Check sheet for the modelled part. Datum: model origin and axes. Units: mm. Face numbers are marked on the shaded views. A direction names the side the tool comes from. Round coordinates to 2 decimals unless told otherwise and drop trailing zeros. Write each loop counter-clockwise with the first axis right and the second up, starting at its lowest first coordinate (ties: lowest second). Pieces come first, ordered by that corner, then holes. Notation, with made-up numbers: (23, 0.5) -> (40, 0.5) arc R18 cw to (40, 14.5) -> close; hole circle Ø1 at (-23, 43). An arc over 180 degrees is marked (long way). One line per item, written item: value.
Autodesk Inventor part; units mm, degrees
ref_plane "YZ Plane" through (0, 0, 0) normal (1, 0, 0) x (0, 1, 0)
ref_plane "XZ Plane" through (0, 0, 0) normal (0, 1, 0) x (-1, 0, 0)
ref_plane "XY Plane" through (0, 0, 0) normal (0, 0, 1) x (1, 0, 0)
sketch "Sketch1" plane through (0, 0, 0) normal (0, 1, 0) x (-1, 0, 0)
  line L0 (50.8, 37.1061) -> (-50.8, 37.1061)
  line L1 (-50.8, 37.1061) -> (-50.8, -37.1061)
  line L2 (-50.8, -37.1061) -> (50.8, -37.1061)
  line L3 (50.8, -37.1061) -> (50.8, 37.1061)
  line L4 (50.8, 37.1061) -> (-50.8, -37.1061) construction
  line L5 (-50.8, 37.1061) -> (50.8, -37.1061) construction
  point P0 (0, 0)
  dimension "d0" = 101.6
  dimension "d1" = 74.2122
extrude "Extrusion1" add sketch "Sketch1" along normal blind 6.35
sketch "Sketch2" plane through (0, 6.35, 0) normal (0, 1, 0) x (1, 0, 0)
  line L0 (-9.525, -19.05) -> (9.525, -19.05)
  line L1 (9.525, -19.05) -> (9.525, 19.05)
  line L2 (9.525, 19.05) -> (-9.525, 19.05)
  line L3 (-9.525, 19.05) -> (-9.525, -19.05)
  line L4 (-9.525, -19.05) -> (9.525, 19.05) construction
  line L5 (9.525, -19.05) -> (-9.525, 19.05) construction
  line L6 (-6.35, -15.875) -> (6.35, -15.875)
  line L7 (6.35, -15.875) -> (6.35, 15.875)
  line L8 (6.35, 15.875) -> (-6.35, 15.875)
  line L9 (-6.35, 15.875) -> (-6.35, -15.875)
  line L10 (-6.35, -15.875) -> (6.35, 15.875) construction
  line L11 (6.35, -15.875) -> (-6.35, 15.875) construction
  point P0 (0, 0)
  dimension "d4" = 19.05
  dimension "d5" = 38.1
  dimension "d6" = 3.175
  dimension "d7" = 3.175
extrude "Extrusion2" add sketch "Sketch2" along normal blind 181.5338
sketch "Sketch3" plane through (9.525, 6.35, 19.05) normal (1, 0, 0) x (0, 0, -1)
  circle A0 centre (19.05, 87.376) radius 4.7625
  line L0 (0, 181.5338) -> (38.1, 181.5338)
  line L1 (-18.0561, 0) -> (56.1561, 0)
  point P0 (19.05, -6.35)
  dimension "d10" = 9.525
  dimension "d14" = 87.376
extrude "Extrusion3" cut sketch "Sketch3" against normal through all
equation "\"d0\" = baseWidth"
equation "\"d2\" = baseThickness"
equation "\"d4\" = postWidth"
equation "\"d5\" = postLength"
equation "\"d6\" = postWallThickness"
equation "\"d7\" = postWallThickness"
equation "\"d8\" = postHeight"
equation "\"d10\" = axelDiam"
equation "\"baseWidth\" = 101.6"
equation "\"baseLength\" = 101.6"
equation "\"baseThickness\" = 6.35"
equation "\"postWidth\" = 19.05"
equation "\"postLength\" = 38.1"
equation "\"postWallThickness\" = 3.175"
equation "\"axelDiam\" = 9.525"
equation "\"distanceFromTopToAxel\" = 25.4"
equation "\"heightOfAxelFromAssembly\" = 156.1338"
properties part number "SupportPost"
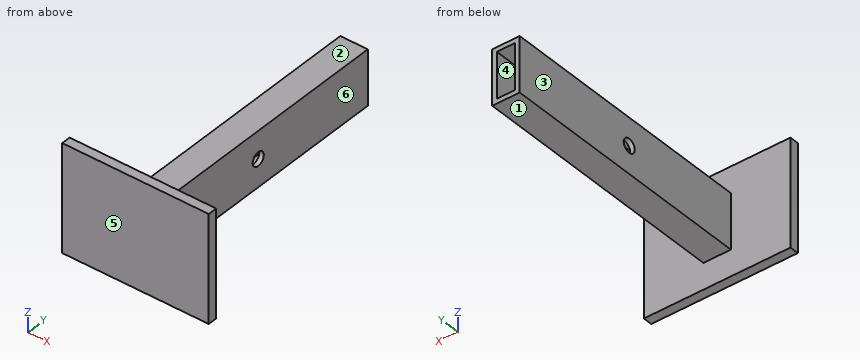
Item 1: Tool access check on the marked faces 1, 2 and 3. Record the directions out of +Z, -Z, +X, -X, +Y, -Y that give a thin tool (end or side, any length) a straight path to the whole face; none if there is none.
Answer:
face 1: -Z, +X, -X, +Y
face 2: +Z, +X, -X, +Y
face 3: +Z, -Z, -X, +Y
Item 2: Sectioned sample at C-C on y = 112. Enter the section's corners in (x, z) (3 decimals), and give its area (3 significant figures).
Answer:
outline: (-9.525, -19.05) -> (9.525, -19.05) -> (9.525, 19.05) -> (-9.525, 19.05) -> close; hole (-6.35, -15.875) -> (6.35, -15.875) -> (6.35, 15.875) -> (-6.35, 15.875) -> close
area: 323 mm^2
Item 3: Sectioned sample at A-A on z = 0. Count the separate pieces of the cut face and the enclosed holes in it, and give its area (3 significant figures).
Answer:
separate pieces: 3
enclosed holes: 0
area: 1,740 mm^2
Item 4: Sectioned sample at B-B on z = 9.5. Enter the section's corners in (x, y) (3 decimals), and give its area (3 significant figures).
Answer:
outline: (-50.8, 0) -> (50.8, 0) -> (50.8, 6.35) -> (9.525, 6.35) -> (9.525, 187.884) -> (6.35, 187.884) -> (6.35, 6.35) -> (-6.35, 6.35) -> (-6.35, 187.884) -> (-9.525, 187.884) -> (-9.525, 6.35) -> (-50.8, 6.35) -> close
area: 1,800 mm^2
Item 5: Sectioned sample at D-D on x = -38. Enter the section's corners in (y, z), and give its area (3 significant figures).
Answer:
outline: (0, -37.11) -> (6.35, -37.11) -> (6.35, 37.11) -> (0, 37.11) -> close
area: 471 mm^2
Item 6: Thickness scan on line 1 (X direction, y = 164.5, z = -1) (3 decimals); line 2 (Z direction, x = 1, y = 78) (3 decimals); line 3 (Y direction, x = -8.5, z = 0). Record the ranges inside material, lowest first.
Answer:
line 1: x = -9.525 to -6.35, 6.35 to 9.525
line 2: z = -19.05 to -15.875, 15.875 to 19.05
line 3: y = 0 to 88.96, 98.49 to 187.88
Item 7: Depth check by flat-ended pin: P1, Ø1.5, axis at x = 20.5, z = -14, coming from the +Y side; P2, Ø14, axis at x = 0, z = -7.5, coming from the +Y side; P3, Ø21, axis at x = 1.5, y = 89, coming from the +Z side; P4, Ø10, axis at y = 60.5, z = -19.5, coming from the -X side (3 decimals). Enter the tip coordinate at first touch or a pass-through.
Answer:
P1: stops at y = 6.35
P2: stops at y = 187.88
P3: stops at z = 19.05
P4: stops at x = -9.525
Item 8: Mould release check, pull along X, two halves, no side actions. Record for the marked faces 4, 5 and 6: pulls with the +X half, pulls with the -X half, needs draft (parallel to the pull), parting line crosses it, or undercut.
Answer:
face 4: undercut
face 5: needs draft
face 6: pulls with the +X half
